Part model, mm, in its own coordinate system. Face numbers are marked on the shaded views. A direction names the side the tool comes from. Round coordinates to 2 decimals unless told otherwise and drop trailing zeros. Write each loop counter-clockwise with the first axis right and the second up, starting at its lowest first coordinate (ties: lowest second). Pieces come first, ordered by that corner, then holes. Notation, with made-up numbers: M 62,-26.75 L 92,-26.75 A14 cw 92,-8.75 Z; hole C 59,62.25 d1. An arc over 180 degrees is marked long. Use one line per item in the form item = value. Start each with the question number.
Item 1: Cut at B-B, the plane y = 8.5. Give the cut face in (x, z), then the cut area to 3 significant figures.
Item 2: Flat gauge pins, fed straight in: pin 1 Ø1.5 at (x, z) = (10, 3) entering from -Y; pin 2 Ø4 at (x, y) = (8.5, 4.5) entering from -Z; pin 3 Ø1.2 at (x, z) = (6.5, 3.5) entering from -Y. Where does each tip first touch, or does it go through?
Item 3: Cut at C-C, the plane x = 9.5. Give the cut face in (y, z).
Item 4: Mould opens along Y. For the marked faces 1, 2 and 3 say: +Y half, -Y half, draft (parallel to the pull), parting line (faces both ways), or undercut.
Item 5: Cut at D-D, the plane y = 11. Give the cut face in (x, z), then the cut area to 3 significant figures.
Item 6: Which spindle directions (+Z, -Z, +X, -X, +Y, -Y) get a long thin tool onto all of the face, cutting with end or side? Do the marked faces 4, 5 and 6. Say none if no direction does.
Item 7: Probe L1, parallel to X at y = 3.5, z = 2.4; L2, parallel to X at y = 5.5, z = 1.65; L3, parallel to X at y = 11.75, z = 0.2. List the from-to ranges inside material, lowest first.
from build123d import *

# Parameters (mm, degrees)
BOSS_EXTRUDE1_DEPTH   = 1.5
BOSS_EXTRUDE1_2_DEPTH = 1.5
BOSS_EXTRUDE2_DEPTH   = 3
FILLET1_R             = 1
SKETCH3_R             = 0.75
CUT_EXTRUDE2_DEPTH    = 29.346075566
FILLET2_R             = 0.5


with BuildPart() as part:
    # Sketch1 → Boss-Extrude1 (new body)
    with BuildSketch(Plane.XY):
        with BuildLine():
            Line((2, 0), (5.3, 0))
            Line((5.3, 0), (5.3, 1))
            Line((5.3, 1), (3.7, 1))
            Line((3.7, 1), (3.7, 3.7))
            Line((3.7, 3.7), (1, 3.7))
            Line((1, 3.7), (1, 14))
            Line((1, 14), (4.5, 14))
            Line((4.5, 14), (4.5, 17.5))
            Line((4.5, 17.5), (5.3, 17.5))
            Line((5.3, 17.5), (5.3, 18.5))
            Line((5.3, 18.5), (2, 18.5))
            ThreePointArc((2, 18.5), (0.585786438, 17.914213562), (0, 16.5))
            Line((0, 16.5), (0, 2))
            ThreePointArc((0, 2), (0.585786438, 0.585786438), (2, 0))
        make_face()
    extrude(amount=BOSS_EXTRUDE1_DEPTH)



with BuildPart() as body_2:
    # Sketch1 → Boss-Extrude1 2 (new body)
    with BuildSketch(Plane.XY):
        with BuildLine():
            Line((21, 2), (21, 16.5))
            ThreePointArc((21, 16.5), (20.414213562, 17.914213562), (19, 18.5))
            Line((19, 18.5), (15.7, 18.5))
            Line((15.7, 18.5), (15.7, 17.5))
            Line((15.7, 17.5), (16.5, 17.5))
            Line((16.5, 17.5), (16.5, 14))
            Line((16.5, 14), (20, 14))
            Line((20, 14), (20, 2))
            ThreePointArc((20, 2), (19.707106781, 1.292893219), (19, 1))
            Line((19, 1), (15.7, 1))
            Line((15.7, 1), (15.7, 0))
            Line((15.7, 0), (19, 0))
            ThreePointArc((19, 0), (20.414213562, 0.585786438), (21, 2))
        make_face()
    extrude(amount=BOSS_EXTRUDE1_2_DEPTH)


with BuildPart() as part_1:
    add(part.part)

    add(body_2.part)  # Boss-Extrude2 merges body 2
    # Sketch2 → Boss-Extrude2 (add)
    with BuildSketch(Plane.XY.offset(1.5)):
        with BuildLine():
            Line((19, 18.5), (15.7, 18.5))
            Line((15.7, 18.5), (15.7, 14))
            Line((15.7, 14), (5.3, 14))
            Line((5.3, 14), (5.3, 18.5))
            Line((5.3, 18.5), (2, 18.5))
            ThreePointArc((2, 18.5), (0.585786438, 17.914213562), (0, 16.5))
            Line((0, 16.5), (0, 2))
            ThreePointArc((0, 2), (0.585786438, 0.585786438), (2, 0))
            Line((2, 0), (5.3, 0))
            Line((5.3, 0), (5.3, 3.7))
            Line((5.3, 3.7), (4.1, 3.7))
            Line((4.1, 3.7), (4.1, 10.2))
            Line((4.1, 10.2), (8.4, 10.2))
            Line((8.4, 10.2), (8.4, 4.5))
            Line((8.4, 4.5), (15.7, 4.5))
            Line((15.7, 4.5), (15.7, 0))
            Line((15.7, 0), (19, 0))
            ThreePointArc((19, 0), (20.414213562, 0.585786438), (21, 2))
            Line((21, 2), (21, 16.5))
            ThreePointArc((21, 16.5), (20.414213562, 17.914213562), (19, 18.5))
        make_face()
    extrude(amount=BOSS_EXTRUDE2_DEPTH)

    # Fillet1
    fillet1_edges = [part_1.edges().sort_by_distance(p)[0] for p in [
        (15.7, 14, 3),
        (5.3, 14, 3),
        (4.1, 3.7, 3),
        (4.1, 10.2, 3),
        (8.4, 10.2, 3),
        (15.7, 4.5, 3),
    ]]
    fillet(fillet1_edges, radius=FILLET1_R)

    # Sketch3 → Cut-Extrude2 (cut, through all)
    with BuildSketch(Plane.XY.offset(4.5)):
        with Locations((9.898564471, 6.065663219)):
            Circle(SKETCH3_R)
        with Locations((5.3005196, 12.837006018)):
            Circle(SKETCH3_R)
        with Locations((16, 15.15)):
            Circle(SKETCH3_R)
    extrude(amount=-CUT_EXTRUDE2_DEPTH, mode=Mode.SUBTRACT)

    # Fillet2
    fillet2_edges = [part_1.edges().sort_by_distance(p)[0] for p in [
        (15.581422532, 14.527671386, 3),
        (15.7, 15.837386354, 3),
    ]]
    fillet(fillet2_edges, radius=FILLET2_R)


solid = part_1.part
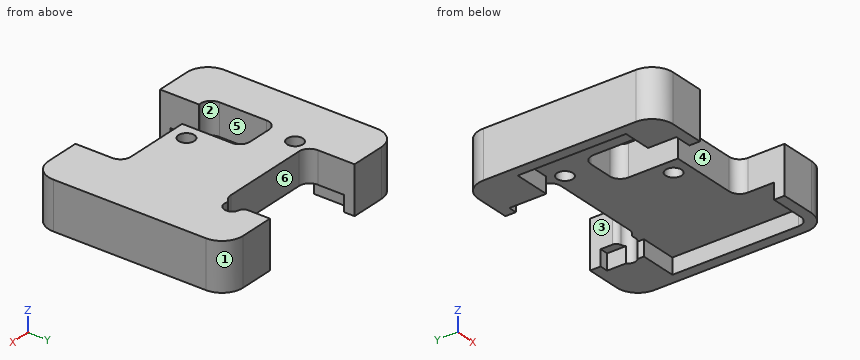
Model answer:
q1.outline = M 0,0 L 1,0 L 1,1.5 L 4.1,1.5 L 4.1,4.5 L 0,4.5 Z; M 8.4,1.5 L 20,1.5 L 20,0 L 21,0 L 21,4.5 L 8.4,4.5 Z
q1.area = 53.1 mm²
q2.pin_1 = 4.5
q2.pin_2 = 1.5
q2.pin_3 = 10.2
q3.outline = M 4.5,1.5 L 5.43,1.5 L 5.43,4.5 L 4.5,4.5 Z; M 6.7,1.5 L 14,1.5 L 14,4.5 L 6.7,4.5 Z
q4.face_1 = +Y half
q4.face_2 = undercut
q4.face_3 = draft
q5.outline = M 0,0 L 1,0 L 1,1.5 L 20,1.5 L 20,0 L 21,0 L 21,4.5 L 0,4.5 Z
q5.area = 66.0 mm²
q6.face_4 = +Z, -Z, -Y
q6.face_5 = +Z, -Z
q6.face_6 = +Z, -Z, +Y
q7.L1 = 0 to 5.3, 15.7 to 21
q7.L2 = 0 to 4.1, 8.4 to 9.41, 10.39 to 21
q7.L3 = 0 to 1, 20 to 21
